Geometry check sheet. Reference: the model listing, model coordinates, mm. A direction names the side the tool comes from. Give positions to 0.01 mm unless a question says otherwise; leave off trailing zeros. Loops run counter-clockwise (first coordinate to the right, second up) from the corner with the lowest first, then second, coordinate; pieces in that order, holes last. Notation, with made-up numbers: (-27.75, -5.75) -> (-12.75, -5.75) arc R18 ccw to (-12.75, 18.25) -> close; hole circle Ø1 at (-21, 74.25). An arc over 180 degrees is marked (long way). Write each question's results on one line, items separated by ' | '. Start each with the question number.
1) Draft check along X on faces 1 (the face through (-26, 44, 0)), 2 (the face through (23.5, 22, 4)), 3 (the face through (0, 2, 16)), 4 (the face through (27.5, 22, 4)). Enter one of: pulls with the +X half, pulls with the -X half, needs draft (parallel to the pull), parting line crosses it, or undercut.
2) Sectioned sample at D-D on y = 5.5. Record the cut outline in (x, z).
3) Sectioned sample at B-B on y = 16.5. Record the cut outline in (x, z), then the cut area to 3 significant figures.
4) Sectioned sample at A-A on x = -2.5. Record the cut outline in (y, z), then the cut area to 3 significant figures.
5) Depth check by flat-ended pin: pin 1 (3 mm diameter, centred on x = 11.5, z = -18.5, fed in from +Y); pin 2 (19 mm diameter, centred on y = 16.5, z = 0, fed in from -X). Enter the tip coordinate at first touch or a pass-through.
6) Sectioned sample at C-C on z = 0. Record the cut outline in (x, y), then the cut area to 3 significant figures.
7) Scan lines: line 1 (X direction, y = 13, z = -10); line 2 (Y direction, x = 26, z = 0); line 3 (Z direction, x = -7, y = 2). Record each from-to range of solid material in increasing order. Write a range as from..to.
8) Set-up check for faces 5 (the face through (25.528, 21.559, 3.226)), 6 (the face through (0, 2, -16)), 7 (the face through (0, 4, -18)): record each of +Z, -Z, +X, -X, +Y, -Y from which the full face is reachable in a straight line by a thin tool's end or side.
```python
from build123d import *

# Parameters (mm, degrees)
SKETCH1_W           = 27.5
SKETCH1_H           = 40
BOSS_EXTRUDE4_DEPTH = 4
SKETCH5_W           = 4
SKETCH5_H           = 40
BOSS_EXTRUDE5_DEPTH = 20
SKETCH6_R           = 6
CUT_EXTRUDE2_DEPTH  = 42.620307543
BOSS_EXTRUDE6_DEPTH = 4
SKETCH8_W           = 47
SKETCH8_H           = 32
CUT_EXTRUDE3_DEPTH  = 53.5


with BuildPart() as part:
    # Sketch1 → Boss-Extrude4 (new body)
    with BuildSketch(Plane(origin=(0, 0, 0), x_dir=(1, 0, 0), z_dir=(0, 1, 0))):
        with Locations((-13.75, 0)):
            Rectangle(SKETCH1_W, SKETCH1_H)
    boss_extrude4 = extrude(amount=BOSS_EXTRUDE4_DEPTH)

    # Sketch5 → Boss-Extrude5 (add)
    with BuildSketch(Plane(origin=(0, 4, 0), x_dir=(1, 0, 0), z_dir=(0, 1, 0))):
        with Locations((-25.5, 0)):
            Rectangle(SKETCH5_W, SKETCH5_H)
    boss_extrude5 = extrude(amount=BOSS_EXTRUDE5_DEPTH)

    # Sketch6 → Cut-Extrude2 (cut, through all)
    with BuildSketch(Plane.ZY.offset(27.5)):
        with Locations((0, 16.5)):
            Circle(SKETCH6_R)
    cut_extrude2 = extrude(amount=-CUT_EXTRUDE2_DEPTH, mode=Mode.SUBTRACT)

    # Sketch7 → Boss-Extrude6 (add)
    with BuildSketch(Plane.ZY.offset(27.5)):
        with BuildLine():
            Line((-20, 24), (20, 24))
            ThreePointArc((20, 24), (0, 44), (-20, 24))
        make_face()
    boss_extrude6 = extrude(amount=-BOSS_EXTRUDE6_DEPTH)

    # Mirror2: Boss-Extrude4, Boss-Extrude5, Cut-Extrude2, Boss-Extrude6 across plane
    add(boss_extrude4.mirror(Plane(origin=(0, 0, 0), x_dir=(0, 0, 1), z_dir=(1, 0, 0))))
    add(boss_extrude5.mirror(Plane(origin=(0, 0, 0), x_dir=(0, 0, 1), z_dir=(1, 0, 0))))
    add(cut_extrude2.mirror(Plane(origin=(0, 0, 0), x_dir=(0, 0, 1), z_dir=(1, 0, 0))), mode=Mode.SUBTRACT)
    add(boss_extrude6.mirror(Plane(origin=(0, 0, 0), x_dir=(0, 0, 1), z_dir=(1, 0, 0))))

    # Sketch8 → Cut-Extrude3 (cut, through all)
    with BuildSketch(Plane(origin=(0, 4, 0), x_dir=(1, 0, 0), z_dir=(0, 1, 0))):
        Rectangle(SKETCH8_W, SKETCH8_H)
    extrude(amount=-CUT_EXTRUDE3_DEPTH, mode=Mode.SUBTRACT)


solid = part.part
```
Result:
1) face 1: needs draft | face 2: undercut | face 3: undercut | face 4: pulls with the +X half
2) outline: (-27.5, -20) -> (-23.5, -20) -> (-23.5, 20) -> (-27.5, 20) -> close; (23.5, -20) -> (27.5, -20) -> (27.5, 20) -> (23.5, 20) -> close
3) outline: (-27.5, -20) -> (-23.5, -20) -> (-23.5, -6) -> (-27.5, -6) -> close; (-27.5, 6) -> (-23.5, 6) -> (-23.5, 20) -> (-27.5, 20) -> close; (23.5, -20) -> (27.5, -20) -> (27.5, -6) -> (23.5, -6) -> close; (23.5, 6) -> (27.5, 6) -> (27.5, 20) -> (23.5, 20) -> close | area: 224 mm^2
4) outline: (0, -20) -> (4, -20) -> (4, -16) -> (0, -16) -> close; (0, 16) -> (4, 16) -> (4, 20) -> (0, 20) -> close | area: 32.0 mm^2
5) pin 1: y = 4 | pin 2: x = -27.5
6) outline: (-27.5, 0) -> (-23.5, 0) -> (-23.5, 10.5) -> (-27.5, 10.5) -> close; (-27.5, 22.5) -> (-23.5, 22.5) -> (-23.5, 44) -> (-27.5, 44) -> close; (23.5, 0) -> (27.5, 0) -> (27.5, 10.5) -> (23.5, 10.5) -> close; (23.5, 22.5) -> (27.5, 22.5) -> (27.5, 44) -> (23.5, 44) -> close | area: 256 mm^2
7) line 1: -27.5..-23.5, 23.5..27.5 | line 2: 0..10.5, 22.5..44 | line 3: -20..-16, 16..20
8) face 5: +X, -X | face 6: +Y, -Y | face 7: +Z, -Z, +Y
